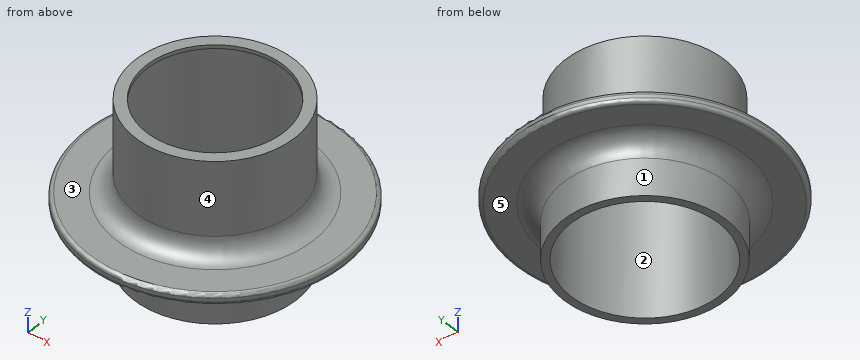
from build123d import *

# Parameters (mm, degrees)
SKETCH_1_R          = 35
EXTRUDE_1_DEPTH     = 43
SKETCH_2_R          = 35
SKETCH_2_R_2        = 22
CUT_EXTRUDE_1_DEPTH = 15
SKETCH_3_R          = 35
SKETCH_3_R_2        = 21.5
CUT_EXTRUDE_2_DEPTH = 25
SKETCH_4_R          = 18.5
CUT_EXTRUDE_3_DEPTH = 44
SKETCH_5_R          = 20
CUT_EXTRUDE_4_DEPTH = 42
FILLET_1_R          = 5
FILLET_2_R          = 1


with BuildPart() as part:
    # ｽｹｯﾁ1 → ﾎﾞｽ - 押し出し1 (new body)
    with BuildSketch(Plane.XY):
        Circle(SKETCH_1_R)
    extrude(amount=EXTRUDE_1_DEPTH)

    # ｽｹｯﾁ2 → ｶｯﾄ - 押し出し1 (cut)
    with BuildSketch(Plane(origin=(0, 0, 0), x_dir=(-1, 0, 0), z_dir=(0, 0, -1))):
        Circle(SKETCH_2_R)
        Circle(SKETCH_2_R_2, mode=Mode.SUBTRACT)
    extrude(amount=-CUT_EXTRUDE_1_DEPTH, mode=Mode.SUBTRACT)

    # ｽｹｯﾁ3 → ｶｯﾄ - 押し出し2 (cut)
    with BuildSketch(Plane.XY.offset(43)):
        Circle(SKETCH_3_R)
        Circle(SKETCH_3_R_2, mode=Mode.SUBTRACT)
    extrude(amount=-CUT_EXTRUDE_2_DEPTH, mode=Mode.SUBTRACT)

    # ｽｹｯﾁ4 → ｶｯﾄ - 押し出し3 (cut, through all)
    with BuildSketch(Plane(origin=(0, 0, 0), x_dir=(-1, 0, 0), z_dir=(0, 0, -1))):
        Circle(SKETCH_4_R)
    extrude(amount=-CUT_EXTRUDE_3_DEPTH, mode=Mode.SUBTRACT)

    # ｽｹｯﾁ5 → ｶｯﾄ - 押し出し4 (cut)
    with BuildSketch(Plane(origin=(0, 0, 0), x_dir=(-1, 0, 0), z_dir=(0, 0, -1))):
        Circle(SKETCH_5_R)
    extrude(amount=-CUT_EXTRUDE_4_DEPTH, mode=Mode.SUBTRACT)

    # ﾌｨﾚｯﾄ1
    fillet_1_edges = [part.edges().sort_by_distance(p)[0] for p in [
        (-21.5, 0, 18),
        (22, 0, 15),
    ]]
    fillet(fillet_1_edges, radius=FILLET_1_R)

    # ﾌｨﾚｯﾄ2
    fillet_2_edges = [part.edges().sort_by_distance(p)[0] for p in [
        (-35, 0, 18),
        (-35, 0, 15),
    ]]
    fillet(fillet_2_edges, radius=FILLET_2_R)


solid = part.part
Here's how the part is built. I have some questions about the finished solid (model axes, mm). Face numbers are marked on the shaded views. A direction names the side the tool comes from. Coordinates: 2 decimals unless noted, no trailing zeros. Order: outer loops, then holes, each group sorted by start corner. A loop starts at its lowest first (then second) coordinate and runs counter-clockwise, first axis right, second up. Notation, with made-up numbers: M 82.5,17 L 131.5,17 A30 ccw 131.5,55 Z; hole C 69,-0.5 d3. An arc over 180 degrees is marked long. Answer as CSV lines item,"result". Start each with the question number.
1. I want a section at A-A, the plane y = 0. Write out the boundary of the cut face in (x, z).
2. For pin 1 (22 mm diameter, centred on x = 0, y = 0, fed in from -Z); pin 2 (1 mm diameter, centred on x = -4.5, z = 35, fed in from +Y); pin 3 (10 mm diameter, centred on x = -14.5, z = 23.5, fed in from -Y); pin 4 (12 mm diameter, centred on y = -22, z = 18.5, fed in from +X), each with a flat end and sliding along its axis, tell me the tip position at first contact or that it passes through.
3. I want a section at C-C, the plane z = 25. Write out the boundary of the cut face in (x, y).
4. We'd pull the mould along Y, two halves only. Please class the marked faces 1, 2 and 3: released by +Y, released by -Y, zero draft, split by the parting line, or undercut.
5. I want a section at D-D, the plane z = 8. Write out the boundary of the cut face in (x, y), and give its area (3 significant figures).
6. On a 3-axis mill with a long thin cutter (end or side, diameter ignored), from which of +Z, -Z, +X, -X, +Y, -Y can I reach the whole of each face in a straight line? I mean the marked faces 4 and 5. Say none if no direction works.
7. I need wall thicknesses on line 1 (Y direction, x = 0, z = 25); line 2 (Y direction, x = 0, z = 42.35); line 3 (X direction, y = 16, z = 6). Which ranges of each line are inside material? Lowest first, please. Write a range as [from, to].
Recorded:
1,outline,"M -35,16 A1 ccw -34,15 L -27,15 A5 cw -22,10 L -22,0 L -20,0 L -20,42 L -18.5,42 L -18.5,43 L -21.5,43 L -21.5,23 A5 cw -26.5,18 L -34,18 A1 ccw -35,17 Z; M 18.5,42 L 20,42 L 20,0 L 22,0 L 22,10 A5 cw 27,15 L 34,15 A1 ccw 35,16 L 35,17 A1 ccw 34,18 L 26.5,18 A5 cw 21.5,23 L 21.5,43 L 18.5,43 Z"
2,pin 1,"passes through"
2,pin 2,"stops at y = 21.12"
2,pin 3,"stops at y = -20.05"
2,pin 4,"stops at x = 31.04"
3,outline,"C 0,0 d43; hole C 0,0 d40"
4,face 1,"split by the parting line"
4,face 2,"undercut"
4,face 3,"zero draft"
5,outline,"C 0,0 d44; hole C 0,0 d40"
5,area,"264 mm2"
6,face 4,"+Z"
6,face 5,"-Z"
7,line 1,"y = [-21.5, -20], [20, 21.5]"
7,line 2,"y = [-21.5, -18.5], [18.5, 21.5]"
7,line 3,"x = [-15.1, -12], [12, 15.1]"
